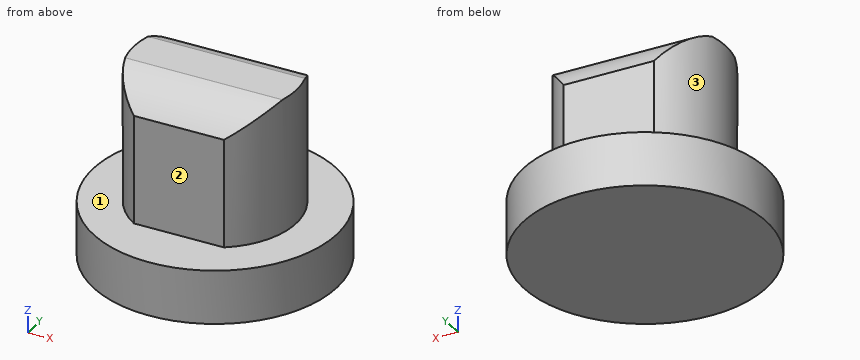
```python
from build123d import *

# Parameters (mm, degrees)
SKETCH_R          = 4.5
PAD_DEPTH         = 2
PAD001_DEPTH      = 7
POCKET_DEPTH      = 4.501
POCKET_DEPTH_BACK = -4.501


with BuildPart() as part:
    # Sketch → Pad (new body)
    with BuildSketch(Plane.XY):
        Circle(SKETCH_R)
    extrude(amount=PAD_DEPTH)

    # Sketch001 → Pad001 (join)
    with BuildSketch(Plane.XY):
        with BuildLine():
            ThreePointArc((-1.658312, 2.5), (-3, 0), (-1.658312, -2.5))
            Line((-1.658312, -2.5), (1.658312, -2.5))
            ThreePointArc((1.658312, -2.5), (3, 0), (1.658312, 2.5))
            Line((-1.658312, 2.5), (1.658312, 2.5))
        make_face()
    extrude(amount=PAD001_DEPTH)

    # Sketch002 → Pocket (cut, two sides)
    with BuildSketch(Plane.YZ) as pocket_sk:
        with BuildLine():
            ThreePointArc((2.746163, 4.734229), (1.500773, 6.674426), (-0.781849, 6.998461))
            ThreePointArc((-0.781849, 6.998461), (-1.981292, 6.473003), (-2.90242, 5.542254))
            Line((-4.129342, 5.542254), (-2.90242, 5.542254))
            Line((-4.129342, 6.557363), (-4.129342, 5.542254))
            Line((-4.129342, 8.966747), (-4.129342, 6.557363))
            Line((2.746163, 8.966747), (-4.129342, 8.966747))
            Line((2.746163, 4.734229), (2.746163, 8.966747))
        make_face()
    extrude(amount=-POCKET_DEPTH, mode=Mode.SUBTRACT)
    extrude(pocket_sk.sketch, amount=-POCKET_DEPTH_BACK, mode=Mode.SUBTRACT)


solid = part.part
```
Check sheet for the modelled part. Datum: model origin and axes. Units: mm. Face numbers are marked on the shaded views. A direction names the side the tool comes from. Round coordinates to 2 decimals unless told otherwise and drop trailing zeros. Loops run counter-clockwise (first coordinate to the right, second up) from the corner with the lowest first, then second, coordinate; pieces in that order, holes last. Notation, with made-up numbers: (-4, 70.5) - (26, 70.5) arc R31 cw to (26, 97.5) - close; hole circle Ø9 at (-9.75, 9). An arc over 180 degrees is marked (long way). Write item = value, one per line. Start each with the question number.
Q1. Access from +Z, -Z, +X, -X, +Y, -Y to the whole of each face (thin tool, end or side, straight path). Record for the marked faces 1, 2 and 3.
Q2. Thickness scan on L1, parallel to Y at x = -2.5, z = 3.75; L2, parallel to Y at x = 0.5, z = 4.25; L3, parallel to Z at x = 0.5, y = 3.75. Record the ranges inside material, lowest first.
Q3. Section check D-D (y = 1.25). Record the boundary of the cut face in (x, z).
Q4. Depth check by flat-ended pin: P1, Ø1.5, axis at y = -2.5, z = 6, coming from the -X side; P2, Ø1.5, axis at y = -1.5, z = 1, coming from the +X side; P3, Ø2, axis at y = 0.5, z = 6, coming from the +X side. Enter the tip coordinate at first touch or a pass-through.
Q5. Section check C-C (z = 5). Record the boundary of the cut face in (x, y), plus the area to 3 significant figures.
Q6. Section check B-B (y = 0). Record the boundary of the cut face in (x, z).
Derived:
q1.face_1 = +Z
q1.face_2 = +Z, +X, -X, -Y
q1.face_3 = +Z, -X
q2.L1 = -1.66 to 1.66
q2.L2 = -2.5 to 2.5
q2.L3 = 0 to 2
q3.outline = (-4.32, 0) - (4.32, 0) - (4.32, 2) - (2.73, 2) - (2.73, 6.82) - (-2.73, 6.82) - (-2.73, 2) - (-4.32, 2) - close
q4.P1 = -2.44
q4.P2 = 4.44
q4.P3 = 3
q5.outline = (-1.66, -2.5) - (1.66, -2.5) arc R3 ccw to (1.66, 2.5) - (-1.66, 2.5) arc R3 ccw to start
q5.area = 26.0 mm^2
q6.outline = (-4.5, 0) - (4.5, 0) - (4.5, 2) - (3, 2) - (3, 7) - (-3, 7) - (-3, 2) - (-4.5, 2) - close
